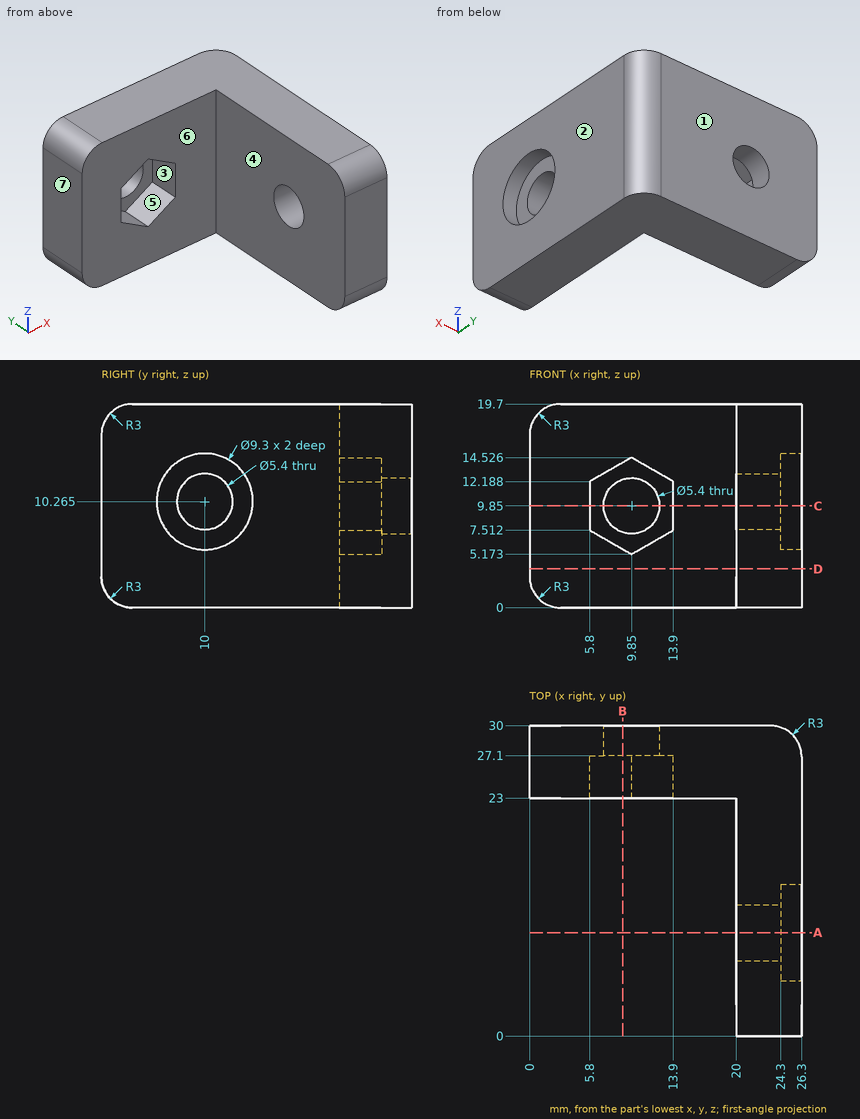
Part print with two shaded views. Sizes in mm from the minimum x, y, z corner. A direction names the side the tool comes from. Round coordinates to 2 decimals unless told otherwise and drop trailing zeros. Write each loop counter-clockwise with the first axis right and the second up, starting at its lowest first coordinate (ties: lowest second). Pieces come first, ordered by that corner, then holes. Notation, with made-up numbers: (85, -27) -> (98, -27) arc R7 cw to (98, -18) -> close; hole circle Ø2 at (10.25, 20). An arc over 180 degrees is marked (long way). Use one line per item in the form item = value.
Q1. Two-plate mould, pull along X, no slides. Class the marked faces 1, 2, 3 and 4: released by +X, released by -X, zero draft, split by the parting line, or undercut.
Conclusion:
face_1 = zero draft
face_2 = released by +X
face_3 = undercut
face_4 = released by -X
Q2. Drop flat-ended pins along their axis: P1, Ø8.5, axis at y = 10, z = 10.265, coming from the -X side; P2, Ø1.5, axis at x = 11, z = 3.5, coming from the -Y side. Give the stop position or say it passes through.
Conclusion:
P1 = 20
P2 = 23
Q3. Drill centre lines: L1, parallel to Z at x = 9.85, y = 28.7; L2, parallel to Y at x = 5.25, z = 17.75; L3, parallel to X at y = 10, z = 17.25. Where is each one in solid material? Low to high.
Conclusion:
L1 = 0 to 7.15, 12.55 to 19.7
L2 = 23 to 30
L3 = 20 to 26.3
Q4. Band-saw the part on B-B, the plane x = 9. Write the cut outline in (y, z) (1 decimal).
Conclusion:
outline = (23, 0) -> (30, 0) -> (30, 7.3) -> (27.1, 7.3) -> (27.1, 5.7) -> (23, 5.7) -> close; (23, 14) -> (27.1, 14) -> (27.1, 12.4) -> (30, 12.4) -> (30, 19.7) -> (23, 19.7) -> close
Q5. Band-saw the part on A-A, the plane y = 10. Write the cut outline in (x, z) (1 decimal).
Conclusion:
outline = (20, 0) -> (26.3, 0) -> (26.3, 5.6) -> (24.3, 5.6) -> (24.3, 7.6) -> (20, 7.6) -> close; (20, 13) -> (24.3, 13) -> (24.3, 14.9) -> (26.3, 14.9) -> (26.3, 19.7) -> (20, 19.7) -> close
Q6. Tool access for the marked faces 5, 6 and 7: list every direction of +Z, -Z, +X, -X, +Y, -Y with a clear straight run to the whole face (end or side of a thin tool).
Conclusion:
face_5 = -Y
face_6 = +Z, -Z, -X, -Y
face_7 = +Z, -Z, -X, +Y, -Y
Q7. Band-saw the part on C-C, the plane z = 9.85. Write the cut outline in (x, y).
Conclusion:
outline = (0, 23) -> (5.8, 23) -> (5.8, 27.1) -> (7.15, 27.1) -> (7.15, 30) -> (0, 30) -> close; (12.55, 27.1) -> (13.9, 27.1) -> (13.9, 23) -> (20, 23) -> (20, 12.67) -> (24.3, 12.67) -> (24.3, 14.63) -> (26.3, 14.63) -> (26.3, 27) arc R3 ccw to (23.3, 30) -> (12.55, 30) -> close; (20, 0) -> (26.3, 0) -> (26.3, 5.37) -> (24.3, 5.37) -> (24.3, 7.33) -> (20, 7.33) -> close
Q8. Band-saw the part on D-D, the plane z = 3.75. Write the cut outline in (x, y).
Conclusion:
outline = (0, 23) -> (20, 23) -> (20, 0) -> (26.3, 0) -> (26.3, 27) arc R3 ccw to (23.3, 30) -> (0, 30) -> close
